```python
from build123d import *

# Parameters (mm, degrees)
SKETCH1_W                 = 19
SKETCH1_H                 = 15.5
BOSS_EXTRUDE1_DEPTH       = 1
F_1_0MM_DOWEL_HOLE1_D     = 2
F_1_0MM_DOWEL_HOLE1_DEPTH = 25
F_1_0MM_DOWEL_HOLE1_TIP   = 0.600860619
SKETCH4_W                 = 15.5
SKETCH4_H                 = 1.015904831
BOSS_EXTRUDE2_DEPTH       = 50


with BuildPart() as part:
    # Sketch1 → Boss-Extrude1 (new body)
    with BuildSketch(Plane(origin=(0, 0, 0), x_dir=(1, 0, 0), z_dir=(0, 1, 0))):
        with Locations((-2.301324503, -0.240066225)):
            Rectangle(SKETCH1_W, SKETCH1_H)
    extrude(amount=BOSS_EXTRUDE1_DEPTH)

    # Ø1.0mm Dowel Hole1
    with Locations(Plane(origin=(0, 1, 0), x_dir=(1, 0, 0), z_dir=(0, 1, 0))):
        with Locations((-6.801324503, 5.259933775), (-6.801324503, -5.740066225)):
            Hole(F_1_0MM_DOWEL_HOLE1_D / 2, depth=F_1_0MM_DOWEL_HOLE1_DEPTH)
            with Locations((0, 0, -(F_1_0MM_DOWEL_HOLE1_DEPTH + F_1_0MM_DOWEL_HOLE1_TIP / 2))):  # 118° drill point
                Cone(0, F_1_0MM_DOWEL_HOLE1_D / 2, F_1_0MM_DOWEL_HOLE1_TIP, mode=Mode.SUBTRACT)

    # Sketch4 → Boss-Extrude2 (add)
    with BuildSketch(Plane(origin=(7.198675497, 0, 0), x_dir=(0, 0, -1), z_dir=(1, 0, 0))):
        with Locations((-0.240066225, 0.492047585)):
            Rectangle(SKETCH4_W, SKETCH4_H)
    extrude(amount=BOSS_EXTRUDE2_DEPTH)


solid = part.part
```
Could you check a few things on this model? Use its own coordinates, in mm. Round coordinates to 2 decimals unless told otherwise and drop trailing zeros.
(1) Thinking about a two-plate mould opening in Z: for faces 1 (the face through (32, -0.016, 0)), 2 (the face through (-7.725, 0.493, -4.877)), which applies, +Z half, -Z half, draft (parallel to the pull), parting line (faces both ways), or undercut?
Findings below:
face 1: draft
face 2: undercut
(2) If I drill on probe 1 along Z at (x, y) = (-6, 0.1); probe 2 along Y at (x, z) = (-7, -6.5); probe 3 along X at (y, z) = (0.6, 6.25), over which ranges is the centre line in solid material (lowest first)?
Findings below:
probe 1: z = -7.51 to -5.86, -4.66 to 5.14, 6.34 to 7.99
probe 2: y = 0 to 1
probe 3: x = -11.8 to -7.66, -5.94 to 57.2
(3) For pin 1 (4.5 mm diameter, centred on x = -1, z = -1, fed in from -Y), with a flat end and sliding along its axis, tell me the tip position at first contact or that it passes through.
Findings below:
pin 1: stops at y = 0
